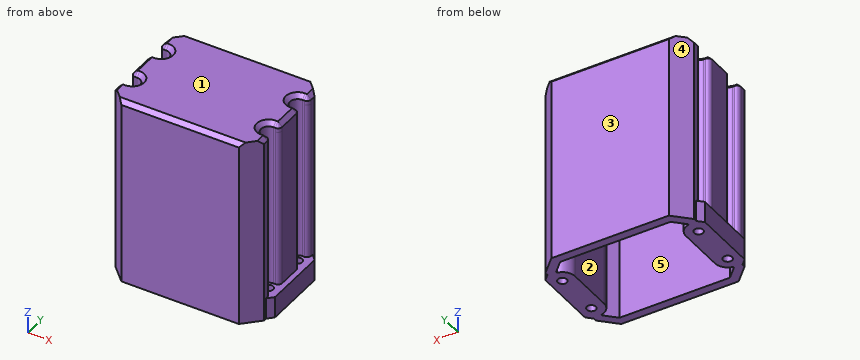
from build123d import *

# Parameters (mm, degrees)
BOSS_EXTRUDE1_DEPTH = 85
SKETCH1_3_R         = 2.125
BOSS_EXTRUDE2_DEPTH = 10
FILLET1_R           = 2
BOSS_EXTRUDE3_START = 4
BOSS_EXTRUDE3_DEPTH = 4
CHAMFER1_SIZE       = 2


with BuildPart() as part:
    # Sketch1 → Boss-Extrude1 (new body)
    with BuildSketch(Plane.XY):
        with BuildLine():
            Line((55.313708499, 53), (0, 53))
            Line((0, 53), (-7.343145751, 45.656854249))
            Line((-7.343145751, 45.656854249), (-7.343145751, 41.125))
            Line((-7.343145751, 41.125), (-4.443145751, 41.125))
            ThreePointArc((-4.443145751, 41.125), (-0.818145751, 37.5), (-4.443145751, 33.875))
            Line((-4.443145751, 33.875), (-7.343145751, 33.875))
            Line((-7.343145751, 33.875), (-7.343145751, 19.125))
            Line((-7.343145751, 19.125), (-4.443145751, 19.125))
            ThreePointArc((-4.443145751, 19.125), (-0.818145751, 15.5), (-4.443145751, 11.875))
            Line((-4.443145751, 11.875), (-7.343145751, 11.875))
            Line((-7.343145751, 11.875), (-7.343145751, 7.343145751))
            Line((-7.343145751, 7.343145751), (0, 0))
            Line((0, 0), (55.313708499, 0))
            Line((55.313708499, 0), (62.656854249, 7.343145751))
            Line((62.656854249, 7.343145751), (62.656854249, 11.875))
            Line((62.656854249, 11.875), (59.756854249, 11.875))
            ThreePointArc((59.756854249, 11.875), (56.131854249, 15.5), (59.756854249, 19.125))
            Line((59.756854249, 19.125), (62.656854249, 19.125))
            Line((62.656854249, 19.125), (62.656854249, 33.875))
            Line((62.656854249, 33.875), (59.756854249, 33.875))
            ThreePointArc((59.756854249, 33.875), (56.131854249, 37.5), (59.756854249, 41.125))
            Line((59.756854249, 41.125), (62.656854249, 41.125))
            Line((62.656854249, 41.125), (62.656854249, 45.656854249))
            Line((62.656854249, 45.656854249), (55.313708499, 53))
        make_face()
        with BuildLine():
            Line((53.656854249, 4), (1.656854249, 4))
            Line((1.656854249, 4), (-3.343145751, 9))
            Line((-3.343145751, 9), (-3.343145751, 9.601695159))
            ThreePointArc((-3.343145751, 9.601695159), (0.172046553, 11.665942097), (1.556854249, 15.5))
            Line((1.556854249, 15.5), (1.556854249, 37.5))
            ThreePointArc((1.556854249, 37.5), (0.172046553, 41.334057903), (-3.343145751, 43.398304841))
            Line((-3.343145751, 43.398304841), (-3.343145751, 44))
            Line((-3.343145751, 44), (1.656854249, 49))
            Line((1.656854249, 49), (53.656854249, 49))
            Line((53.656854249, 49), (58.656854249, 44))
            Line((58.656854249, 44), (58.656854249, 43.398304841))
            ThreePointArc((58.656854249, 43.398304841), (55.141661946, 41.334057903), (53.756854249, 37.5))
            Line((53.756854249, 37.5), (53.756854249, 15.5))
            ThreePointArc((53.756854249, 15.5), (55.141661946, 11.665942097), (58.656854249, 9.601695159))
            Line((58.656854249, 9.601695159), (58.656854249, 9))
            Line((58.656854249, 9), (53.656854249, 4))
        make_face(mode=Mode.SUBTRACT)
    extrude(amount=BOSS_EXTRUDE1_DEPTH)

    # Sketch1<3> → Boss-Extrude2 (add)
    # profile 1 of 2: a face of its own
    with BuildSketch(Plane.XY):
        with BuildLine():
            ThreePointArc((-4.443145751, 33.875), (-0.818145751, 37.5), (-4.443145751, 41.125))
            Line((-4.443145751, 41.125), (-7.343145751, 41.125))
            Line((-7.343145751, 41.125), (-7.343145751, 44.1))
            Line((-7.343145751, 44.1), (-9.943145751, 41.5))
            Line((-9.943145751, 41.5), (-9.943145751, 11.5))
            Line((-9.943145751, 11.5), (-7.343145751, 8.9))
            Line((-7.343145751, 8.9), (-7.343145751, 11.875))
            Line((-7.343145751, 11.875), (-4.443145751, 11.875))
            ThreePointArc((-4.443145751, 11.875), (-0.818145751, 15.5), (-4.443145751, 19.125))
            Line((-4.443145751, 19.125), (-7.343145751, 19.125))
            Line((-7.343145751, 19.125), (-7.343145751, 33.875))
            Line((-7.343145751, 33.875), (-4.443145751, 33.875))
        make_face()
        with Locations((-4.443145751, 15.5)):
            Circle(SKETCH1_3_R, mode=Mode.SUBTRACT)
        with Locations((-4.443145751, 37.5)):
            Circle(SKETCH1_3_R, mode=Mode.SUBTRACT)
    # profile 2 of 2: a face of its own
    with BuildSketch(Plane.XY):
        with BuildLine():
            Line((65.256854249, 41.5), (62.656854249, 44.1))
            Line((62.656854249, 44.1), (62.656854249, 41.125))
            Line((62.656854249, 41.125), (59.756854249, 41.125))
            ThreePointArc((59.756854249, 41.125), (56.131854249, 37.5), (59.756854249, 33.875))
            Line((59.756854249, 33.875), (62.656854249, 33.875))
            Line((62.656854249, 33.875), (62.656854249, 19.125))
            Line((62.656854249, 19.125), (59.756854249, 19.125))
            ThreePointArc((59.756854249, 19.125), (56.131854249, 15.5), (59.756854249, 11.875))
            Line((59.756854249, 11.875), (62.656854249, 11.875))
            Line((62.656854249, 11.875), (62.656854249, 8.9))
            Line((62.656854249, 8.9), (65.256854249, 11.5))
            Line((65.256854249, 11.5), (65.256854249, 41.5))
        make_face()
        with Locations((59.756854249, 37.5)):
            Circle(SKETCH1_3_R, mode=Mode.SUBTRACT)
        with Locations((59.756854249, 15.5)):
            Circle(SKETCH1_3_R, mode=Mode.SUBTRACT)
    extrude(amount=BOSS_EXTRUDE2_DEPTH)

    # Fillet1
    fillet1_edges = [part.edges().sort_by_distance(p)[0] for p in [
        (62.656854249, 41.125, 47.5),
        (62.656854249, 33.875, 47.5),
        (62.656854249, 19.125, 47.5),
        (62.656854249, 11.875, 47.5),
        (-7.343145751, 11.875, 47.5),
        (-7.343145751, 19.125, 47.5),
        (-7.343145751, 33.875, 47.5),
        (-7.343145751, 41.125, 47.5),
    ]]
    fillet(fillet1_edges, radius=FILLET1_R)

    # Sketch2 → Boss-Extrude3 (add)
    with BuildSketch(Plane.XY.offset(85).offset(BOSS_EXTRUDE3_START)):
        with BuildLine():
            Line((-7.343145751, 31.875), (-7.343145751, 21.125))
            ThreePointArc((-7.343145751, 21.125), (-6.757359313, 19.710786438), (-5.343145751, 19.125))
            Line((-5.343145751, 19.125), (-4.443145751, 19.125))
            ThreePointArc((-4.443145751, 19.125), (-0.818145751, 15.5), (-4.443145751, 11.875))
            Line((-4.443145751, 11.875), (-5.343145751, 11.875))
            ThreePointArc((-5.343145751, 11.875), (-6.757359313, 11.289213562), (-7.343145751, 9.875))
            Line((-7.343145751, 9.875), (-7.343145751, 7.343145751))
            Line((-7.343145751, 7.343145751), (0, 0))
            Line((0, 0), (55.313708499, 0))
            Line((55.313708499, 0), (62.656854249, 7.343145751))
            Line((62.656854249, 7.343145751), (62.656854249, 9.875))
            ThreePointArc((62.656854249, 9.875), (62.071067812, 11.289213562), (60.656854249, 11.875))
            Line((60.656854249, 11.875), (59.756854249, 11.875))
            ThreePointArc((59.756854249, 11.875), (56.131854249, 15.5), (59.756854249, 19.125))
            Line((59.756854249, 19.125), (60.656854249, 19.125))
            ThreePointArc((60.656854249, 19.125), (62.071067812, 19.710786438), (62.656854249, 21.125))
            Line((62.656854249, 21.125), (62.656854249, 31.875))
            ThreePointArc((62.656854249, 31.875), (62.071067812, 33.289213562), (60.656854249, 33.875))
            Line((60.656854249, 33.875), (59.756854249, 33.875))
            ThreePointArc((59.756854249, 33.875), (56.131854249, 37.5), (59.756854249, 41.125))
            Line((59.756854249, 41.125), (60.656854249, 41.125))
            ThreePointArc((60.656854249, 41.125), (62.071067812, 41.710786438), (62.656854249, 43.125))
            Line((62.656854249, 43.125), (62.656854249, 45.656854249))
            Line((62.656854249, 45.656854249), (55.313708499, 53))
            Line((55.313708499, 53), (0, 53))
            Line((0, 53), (-7.343145751, 45.656854249))
            Line((-7.343145751, 45.656854249), (-7.343145751, 43.125))
            ThreePointArc((-7.343145751, 43.125), (-6.757359313, 41.710786438), (-5.343145751, 41.125))
            Line((-5.343145751, 41.125), (-4.443145751, 41.125))
            ThreePointArc((-4.443145751, 41.125), (-0.818145751, 37.5), (-4.443145751, 33.875))
            Line((-4.443145751, 33.875), (-5.343145751, 33.875))
            ThreePointArc((-5.343145751, 33.875), (-6.757359313, 33.289213562), (-7.343145751, 31.875))
        make_face()
    extrude(amount=-BOSS_EXTRUDE3_DEPTH)

    # Chamfer1
    chamfer1_edges = [part.edges().sort_by_distance(p)[0] for p in [
        (-7.343145751, 44.390927125, 89),
        (-6.757359313, 41.710786438, 89),
        (-4.893145751, 41.125, 89),
        (-0.818145751, 37.5, 89),
        (-4.893145751, 33.875, 89),
        (-6.757359313, 33.289213562, 89),
        (-7.343145751, 26.5, 89),
        (-6.757359313, 19.710786438, 89),
        (-4.893145751, 19.125, 89),
        (-0.818145751, 15.5, 89),
        (-4.893145751, 11.875, 89),
        (-6.757359313, 11.289213562, 89),
        (-7.343145751, 8.609072875, 89),
        (27.656854249, 0, 89),
        (62.656854249, 8.609072875, 89),
        (62.071067812, 11.289213562, 89),
        (60.206854249, 11.875, 89),
        (56.131854249, 15.5, 89),
        (60.206854249, 19.125, 89),
        (62.071067812, 19.710786438, 89),
        (62.656854249, 26.5, 89),
        (62.071067812, 33.289213562, 89),
        (60.206854249, 33.875, 89),
        (56.131854249, 37.5, 89),
        (60.206854249, 41.125, 89),
        (62.071067812, 41.710786438, 89),
        (62.656854249, 44.390927125, 89),
        (27.656854249, 53, 89),
    ]]
    chamfer(chamfer1_edges, length=CHAMFER1_SIZE - 0.0001)  # a hair under: the kernel refuses the full size


solid = part.part
Work out the finished part from the listing and answer in its coordinate system (mm). Face numbers are marked on the shaded views. A direction names the side the tool comes from. Round coordinates to 2 decimals unless told otherwise and drop trailing zeros. Loops run counter-clockwise (first coordinate to the right, second up) from the corner with the lowest first, then second, coordinate; pieces in that order, holes last. Notation, with made-up numbers: (69.25, 7) - (91.25, 7) arc R6 cw to (91.25, 13) - close; hole circle Ø8 at (-35, -33). An arc over 180 degrees is marked (long way). Use one line per item in the form item = value. Start each with the question number.
(1) Which of the six approach directions +Z, -Z, +X, -X, +Y, -Y give full straight-line access (tool end or side, diameter ignored) to the marked faces 1 and 2?
(2) Consider line 1 (Y direction, x = 51, z = 44); line 2 (Y direction, x = 57.5, z = 65.5); line 3 (X direction, y = 30, z = 65). Determine where each line is inside the solid, lowest interval first.
(3) Find section A-A on x = 22. Determine the outline of the cut face in (y, z).
(4) Flat-ended cylindrical pins translate along their axes: P1, Ø1, axis at x = 24, y = 22.5, coming from the -Z side; P2, Ø5, axis at y = 15, z = 59, coming from the +X side; P3, Ø12, axis at y = 37.5, z = 37, coming from the -X side; P4, Ø3.5, axis at x = 59.76, y = 37.5, coming from the +Z side. Find the tip coordinate at first contact, or state that the pin passes through.
(5) Determine the mould class of the marked faces 3, 4 and 5 for opening direction X: +X half, -X half, draft (parallel to the pull), parting line (faces both ways), or undercut.
Answer list:
q1.face_1 = +Z, +X, -X, +Y, -Y
q1.face_2 = -Z
q2.line_1 = 0 to 4, 49 to 53
q2.line_2 = 2.19 to 7.84, 9.94 to 12.66, 18.34 to 34.66, 40.34 to 43.06, 45.16 to 50.81
q2.line_3 = -7.34 to 1.56, 53.76 to 62.66
q3.outline = (0, 0) - (4, 0) - (4, 85) - (49, 85) - (49, 0) - (53, 0) - (53, 87) - (51, 89) - (2, 89) - (0, 87) - close
q4.P1 = 85
q4.P2 = 57.72
q4.P3 = -7.34
q4.P4 = through
q5.face_3 = draft
q5.face_4 = -X half
q5.face_5 = undercut
